from build123d import *

# Parameters (mm, degrees)
SKETCH1_R                     = 1.5
BOSS_EXTRUDE1_DEPTH           = 2
M3_CLEARANCE_HOLE1_D          = 3
M3_CLEARANCE_HOLE1_DEPTH      = 2
M3_CLEARANCE_HOLE1_TIP        = 0.901290929
BOSS_EXTRUDE2_START           = -2
SKETCH5_R                     = 1.6
BOSS_EXTRUDE2_DEPTH           = 2
CUT_EXTRUDE1_DEPTH            = 2
CUT_EXTRUDE2_START            = -10
SKETCH8_R                     = 96.999999979
SKETCH8_R_2                   = 86.999999979
CUT_EXTRUDE2_DEPTH            = 10
SKETCH10_W                    = 43
SKETCH10_H                    = 109
CUT_EXTRUDE3_DEPTH            = 10
CSK_FOR_M3_SFHCS1_D           = 3
CSK_FOR_M3_SFHCS1_DEPTH       = 9.5
CSK_FOR_M3_SFHCS1_CSINK_D     = 5.6
CSK_FOR_M3_SFHCS1_CSINK_ANGLE = 90
CSK_FOR_M3_SFHCS1_TIP         = 0.901290929
F_3_0_3_DIAMETER_HOLE1_D      = 3
F_3_0_3_DIAMETER_HOLE1_DEPTH  = 3
F_3_0_3_DIAMETER_HOLE1_TIP    = 0.901290929
FILLET1_R                     = 2


with BuildPart() as part:
    # Sketch1 → Boss-Extrude1 (new body)
    with BuildSketch(Plane(origin=(0, 0, 0), x_dir=(-1, 0, 0), z_dir=(0, 0, -1))):
        with BuildLine():
            Line((49.999999993, 72.000000003), (34.499999968, 72.000000003))
            ThreePointArc((34.499999968, 72.000000003), (33.085786407, 71.414213566), (32.49999997, 70.000000005))
            Line((32.49999997, 70.000000005), (32.49999997, 50.749999994))
            ThreePointArc((32.49999997, 50.749999994), (31.914213535, 49.335786439), (30.49999998, 48.750000004))
            Line((30.49999998, 48.750000004), (-30.50000002, 48.750000004))
            ThreePointArc((-30.50000002, 48.750000004), (-31.914213575, 49.335786439), (-32.50000001, 50.749999994))
            Line((-32.50000001, 50.749999994), (-32.50000001, 69.749999994))
            ThreePointArc((-32.50000001, 69.749999994), (-33.085786447, 71.164213555), (-34.500000007, 71.749999992))
            Line((-34.500000007, 71.749999992), (-50.000000007, 71.749999992))
            ThreePointArc((-50.000000007, 71.749999992), (-52.651650433, 70.651650422), (-53.750000002, 67.999999996))
            Line((-53.750000002, 67.999999996), (-53.750000002, 40.749999996))
            ThreePointArc((-53.750000002, 40.749999996), (-53.164213571, 39.335786449), (-51.750000024, 38.750000018))
            Line((-51.750000024, 38.750000018), (-39.000000024, 38.750000018))
            ThreePointArc((-39.000000024, 38.750000018), (-36.171572886, 37.578427137), (-35.000000005, 34.75))
            Line((-35.000000005, 34.75), (-35.000000005, -46))
            ThreePointArc((-35.000000005, -46), (-36.171572879, -48.828427121), (-38.999999999, -49.999999994))
            Line((-38.999999999, -49.999999994), (-45.09502308, -49.999999994))
            ThreePointArc((-45.09502308, -49.999999994), (-54.039294999, -55.527864046), (-53.095023084, -66.000000011))
            ThreePointArc((-53.095023084, -66.000000011), (-46.752677079, -72.686883058), (-39.048234252, -77.744680848))
            ThreePointArc((-39.048234252, -77.744680848), (2e-09, -86.999999997), (39.048234252, -77.744680848))
            ThreePointArc((39.048234252, -77.744680848), (46.752677083, -72.686883063), (53.095023084, -66.000000011))
            ThreePointArc((53.095023084, -66.000000011), (54.039295004, -55.527864051), (45.09502308, -49.999999994))
            Line((45.09502308, -49.999999994), (39.000000001, -49.999999994))
            ThreePointArc((39.000000001, -49.999999994), (36.17157288, -48.828427121), (35.000000007, -46))
            Line((35.000000007, -46), (35.000000007, 34.75))
            ThreePointArc((35.000000007, 34.75), (36.171572888, 37.578427137), (39.000000025, 38.750000018))
            Line((39.000000025, 38.750000018), (51.750000009, 38.750000018))
            ThreePointArc((51.750000009, 38.750000018), (53.164213556, 39.335786449), (53.749999988, 40.749999996))
            Line((53.749999988, 40.749999996), (53.749999988, 68.250000008))
            ThreePointArc((53.749999988, 68.250000008), (52.651650419, 70.901650434), (49.999999993, 72.000000003))
        make_face()
        with Locations((49.348831914, 65.488111827)):
            Circle(SKETCH1_R, mode=Mode.SUBTRACT)
        with Locations((-49.348831883, 65.488111827)):
            Circle(SKETCH1_R, mode=Mode.SUBTRACT)
        with Locations((28.045651768, -77.054794901)):
            Circle(SKETCH1_R, mode=Mode.SUBTRACT)
        with Locations((-28.045651737, -77.054794901)):
            Circle(SKETCH1_R, mode=Mode.SUBTRACT)
    extrude(amount=-BOSS_EXTRUDE1_DEPTH)

    # M3 Clearance Hole1
    with Locations(Plane(origin=(-39.259818305, 68, 2), x_dir=(1, 0, 0), z_dir=(0, 0, 1))):
        with Locations((0, 0), (78.51963661, 0)):
            Hole(M3_CLEARANCE_HOLE1_D / 2, depth=M3_CLEARANCE_HOLE1_DEPTH)
            with Locations((0, 0, -(M3_CLEARANCE_HOLE1_DEPTH + M3_CLEARANCE_HOLE1_TIP / 2))):  # 118° drill point
                Cone(0, M3_CLEARANCE_HOLE1_D / 2, M3_CLEARANCE_HOLE1_TIP, mode=Mode.SUBTRACT)

    # Sketch5 → Boss-Extrude2 (add)
    with BuildSketch(Plane.XY.offset(2).offset(BOSS_EXTRUDE2_START)):
        with BuildLine():
            Line((-48.836461775, 72), (48.836461775, 72))
            ThreePointArc((48.836461775, 72), (0, -86.999999993), (-48.836461775, 72))
        make_face()
        with Locations((-39.259818305, 68)):
            Circle(SKETCH5_R, mode=Mode.SUBTRACT)
        with Locations((39.259818305, 68)):
            Circle(SKETCH5_R, mode=Mode.SUBTRACT)
        with Locations((-28.045651768, -77.054794901)):
            Circle(SKETCH5_R, mode=Mode.SUBTRACT)
        with Locations((28.045651737, -77.054794901)):
            Circle(SKETCH5_R, mode=Mode.SUBTRACT)
    extrude(amount=BOSS_EXTRUDE2_DEPTH)

    # Sketch6 → Cut-Extrude1 (cut)
    with BuildSketch(Plane.XY.offset(2)):
        with BuildLine():
            Line((-75.175409678, -27.361611463), (-40.000000015, -27.361611463))
            Line((-40.000000015, -27.361611463), (-40.000000015, -69.2820323))
            ThreePointArc((-40.000000015, -69.2820323), (-61.283555465, -51.423008772), (-75.175409678, -27.361611463))
        make_face()
        with BuildLine():
            Line((41.568542512, 27.361611478), (75.175409701, 27.361611478))
            ThreePointArc((75.175409701, 27.361611478), (67.471315698, 42.983968695), (56.568542512, 56.568542531))
            Line((56.568542512, 56.568542531), (41.568542512, 56.568542531))
            Line((41.568542512, 56.568542531), (41.568542512, 27.361611478))
        make_face()
        with BuildLine():
            Line((40.000000015, -27.361611463), (40.000000015, -69.2820323))
            ThreePointArc((40.000000015, -69.2820323), (61.283555468, -51.423008776), (75.175409678, -27.361611463))
            Line((75.175409678, -27.361611463), (40.000000015, -27.361611463))
        make_face()
        with BuildLine():
            Line((-56.568542512, 56.568542531), (-41.568542512, 56.568542531))
            Line((-41.568542512, 56.568542531), (-41.568542512, 27.361611478))
            Line((-41.568542512, 27.361611478), (-75.175409701, 27.361611478))
            ThreePointArc((-75.175409701, 27.361611478), (-67.471315695, 42.983968693), (-56.568542512, 56.568542531))
        make_face()
    extrude(amount=-CUT_EXTRUDE1_DEPTH, mode=Mode.SUBTRACT)

    # Sketch8 → Cut-Extrude2 (cut)
    with BuildSketch(Plane.XY.offset(2).offset(CUT_EXTRUDE2_START)):
        Circle(SKETCH8_R)
        Circle(SKETCH8_R_2, mode=Mode.SUBTRACT)
    extrude(amount=CUT_EXTRUDE2_DEPTH, mode=Mode.SUBTRACT)

    # Sketch10 → Cut-Extrude3 (cut)
    with BuildSketch(Plane.XY.offset(2)):
        with Locations((0, -19.499999997)):
            Rectangle(SKETCH10_W, SKETCH10_H)
    extrude(amount=-CUT_EXTRUDE3_DEPTH, mode=Mode.SUBTRACT)

    # CSK for M3 SFHCS1
    with Locations(Plane(origin=(0, 38.500000003, 2), x_dir=(1, 0, 0), z_dir=(0, 0, 1))):
        with Locations((0, 0), (-25, -48), (0, -116), (-79.647661626, -58), (79.647661626, -58), (-43.018232726, 22.936403319), (-28.045651768, -115.554794904), (43.018232726, 22.936403319), (25, -48), (28.045651737, -115.554794904)):
            CounterSinkHole(CSK_FOR_M3_SFHCS1_D / 2, CSK_FOR_M3_SFHCS1_CSINK_D / 2, depth=CSK_FOR_M3_SFHCS1_DEPTH, counter_sink_angle=CSK_FOR_M3_SFHCS1_CSINK_ANGLE)
            with Locations((0, 0, -(CSK_FOR_M3_SFHCS1_DEPTH + CSK_FOR_M3_SFHCS1_TIP / 2))):  # 118° drill point
                Cone(0, CSK_FOR_M3_SFHCS1_D / 2, CSK_FOR_M3_SFHCS1_TIP, mode=Mode.SUBTRACT)

    # Ø3.0 (3) Diameter Hole1
    with Locations(Plane(origin=(-71, 23.5, 2), x_dir=(1, 0, 0), z_dir=(0, 0, 1))):
        with Locations((0, 0), (0, -47), (40, -89.5), (33.318788522, -97.453541508), (40, 42.5), (102, 42.5), (142, 0), (102, -89.5), (142, -47), (108.681211478, -97.453541508)):
            Hole(F_3_0_3_DIAMETER_HOLE1_D / 2, depth=F_3_0_3_DIAMETER_HOLE1_DEPTH)
            with Locations((0, 0, -(F_3_0_3_DIAMETER_HOLE1_DEPTH + F_3_0_3_DIAMETER_HOLE1_TIP / 2))):  # 118° drill point
                Cone(0, F_3_0_3_DIAMETER_HOLE1_D / 2, F_3_0_3_DIAMETER_HOLE1_TIP, mode=Mode.SUBTRACT)

    # Fillet1
    fillet1_edges = [part.edges().sort_by_distance(p)[0] for p in [
        (48.836461775, 72, 1),
        (-40.000000015, -69.2820323, 1),
        (-75.175409678, -27.361611463, 1),
        (-40.000000015, -27.361611463, 1),
        (41.568542512, 27.361611478, 1),
        (41.568542512, 56.568542531, 1),
        (56.568542512, 56.568542531, 1),
        (75.175409701, 27.361611478, 1),
        (40.000000015, -27.361611463, 1),
        (75.175409678, -27.361611463, 1),
        (40.000000015, -69.2820323, 1),
        (-75.175409701, 27.361611478, 1),
        (-56.568542512, 56.568542531, 1),
        (-41.568542512, 56.568542531, 1),
        (-41.568542512, 27.361611478, 1),
        (-48.836461746, 72.000000003, 1),
        (21.5, 35.000000003, 1),
        (21.5, -73.999999997, 1),
        (-21.5, -73.999999997, 1),
        (-21.5, 35.000000003, 1),
    ]]
    fillet(fillet1_edges, radius=FILLET1_R)


solid = part.part
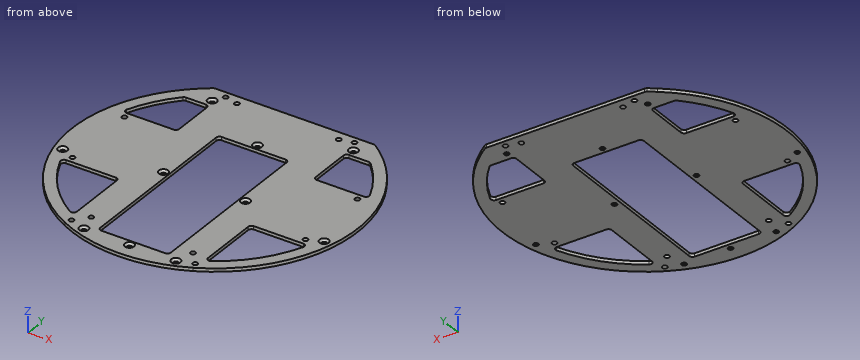
CAD build for the part. Positions are in the model's coordinates, mm. Coordinates: 2 decimals unless noted, no trailing zeros. Order: outer loops, then holes, each group sorted by start corner. A loop starts at its lowest first (then second) coordinate and runs counter-clockwise, first axis right, second up.
Item 1: Band-saw the part on B-B on x = 62. List the corners of the cut face in (y, z), plus the area to 3 significant figures.
Check sheet entries:
outline: (-61.03, 0) - (-50.56, 0) - (-50.56, 2) - (-61.03, 2) - close; (-27.36, 0) - (27.36, 0) - (27.36, 2) - (-27.36, 2) - close; (50.56, 0) - (61.03, 0) - (61.03, 2) - (50.56, 2) - close
area: 151 mm2
Item 2: Drill centre lines: L1, parallel to X at y = -32, z = 0.15; L2, parallel to X at y = 46, z = 1.3; L3, parallel to X at y = 22.5, z = 0.6. Where is each one in solid material? Low to high.
Check sheet entries:
L1: x = -80.9 to -73.32, -40 to -21.5, 21.5 to 40, 73.32 to 80.9
L2: x = -73.84 to -65.45, -41.57 to 41.57, 65.45 to 73.84
L3: x = -84.04 to -72.12, -69.88 to -21.5, 21.5 to 69.88, 72.12 to 84.04
Item 3: Band-saw the part on A-A on x = 9. List the corners of the cut face in (y, z), plus the area to 3 significant figures.
Check sheet entries:
outline: (-86.53, 0) - (-74, 0) - (-74, 2) - (-86.53, 2) - close; (35, 0) - (72, 0) - (72, 2) - (35, 2) - close
area: 99.1 mm2
Item 4: Pin check, flat tips, straight feed: pin 1 Ø1 at (y, z) = (37.5, 0.5) entering from +X; pin 2 Ø2.5 at (x, y) = (0, -77.5) entering from -Z; pin 3 Ø0.6 at (x, z) = (51.5, 0.5) entering from +Y; pin 4 Ø3.5 at (x, y) = (43.02, 61.44) entering from +Z. Stop position of each tip, or through.
Check sheet entries:
pin 1: stops at x = 78.74
pin 2: passes through
pin 3: stops at y = 70.34
pin 4: stops at z = 0.95
Item 5: Band-saw the part on C-C on y = 19.5. List the corners of the cut face in (x, z).
Check sheet entries:
outline: (-84.79, 0) - (-21.5, 0) - (-21.5, 2) - (-84.79, 2) - close; (21.5, 0) - (84.79, 0) - (84.79, 2) - (21.5, 2) - close
Item 6: Band-saw the part on D-D on z = 1.3. Give the number of separate pieces and of enclosed holes in the cut face, plus the area to 3 significant figures.
Check sheet entries:
separate pieces: 1
enclosed holes: 27
area: 14,600 mm2
